Autodesk Inventor part; units mm, degrees
ref_plane "YZ Plane" through (0, 0, 0) normal (1, 0, 0) x (0, 1, 0)
ref_plane "XZ Plane" through (0, 0, 0) normal (0, 1, 0) x (-1, 0, 0)
ref_plane "XY Plane" through (0, 0, 0) normal (0, 0, 1) x (1, 0, 0)
ref_plane "Work Plane1" through (0, 0, -1.5) normal (0, 0, -1) x (-1, 0, 0)
sketch "Sketch1" plane through (0, 0, -1.5) normal (0, 0, -1) x (-1, 0, 0)
  line L0 (11.5, -60) -> (11.5, -65)
  arc A0 (9.3, -67.4819) -> (11.5, -65) centre (9, -65) ccw
  arc A1 (11.5, -60) -> (9.3, -57.5181) centre (9, -60) ccw
  line L1 (15, -75) -> (9.3, -75)
  line L2 (15, -5) -> (15, -75)
  line L3 (9.3, -5) -> (15, -5)
  line L4 (6.75, -60) -> (6.75, -65)
  arc A2 (6.75, -65) -> (11.25, -65) centre (9, -65) ccw
  line L5 (11.25, -65) -> (11.25, -60)
  arc A3 (11.25, -60) -> (6.75, -60) centre (9, -60) ccw
  line L6 (9, -65) -> (9, -61.5) construction
  line L7 (6.75, -65) -> (6.75, -61.5)
  line L8 (11.25, -61.5) -> (11.25, -65)
  arc A4 (6.75, -65) -> (11.25, -65) centre (9, -65) ccw
  arc A5 (11.25, -61.5) -> (6.75, -61.5) centre (9, -61.5) ccw
  line L9 (9.3, -57.5181) -> (9.3, -5)
  line L10 (9.3, -75) -> (9.3, -67.4819)
  point P0 (0, 0)
  point P1 (9, -63.25)
  dimension "d0" = 0.25
  dimension "d1" = 3.5
extrude "Extrusion1" add sketch "Sketch1" along normal blind 0.5 and the other way blind 1.5 contours A5 L5 A2 L4
sketch "Sketch2" plane through (0, 0, 0) normal (0, 0, 1) x (1, 0, 0)
  line L0 (-6.75, -65) -> (-6.75, -61.5)
  arc A0 (-6.75, -61.5) -> (-11.25, -61.5) centre (-9, -61.5) ccw
  line L1 (-11.25, -61.5) -> (-11.25, -65)
  arc A1 (-11.25, -65) -> (-6.75, -65) centre (-9, -65) ccw
  line L2 (-12.5, -69.5) -> (-5.5, -69.5)
  line L3 (-5.5, -69.5) -> (-5.5, -60.5)
  line L4 (-5.5, -60.5) -> (-12.5, -60.5)
  line L5 (-12.5, -60.5) -> (-12.5, -69.5)
  line L6 (-12.5, -69.5) -> (-5.5, -60.5) construction
  line L7 (-5.5, -69.5) -> (-12.5, -60.5) construction
  line L8 (-12.5, -57) -> (-5.5, -57)
  line L9 (-5.5, -57) -> (-5.5, -66)
  line L10 (-5.5, -66) -> (-12.5, -66)
  line L11 (-12.5, -66) -> (-12.5, -57)
  line L12 (-12.5, -57) -> (-5.5, -66) construction
  line L13 (-5.5, -57) -> (-12.5, -66) construction
  point P0 (0, 0)
  dimension "d6" = 7
  dimension "d7" = 7
  dimension "d9" = 9
extrude "Extrusion2" add sketch "Sketch2" along normal blind 1
ref_plane "Work Plane2" through (-10.6833, -67.2, 6.3) normal (-1, 0, 0) x (0, 0, 1)
sketch "Sketch3" plane through (-10.6833, -67.2, 6.3) normal (-1, 0, 0) x (0, 0, 1)
  line L0 (0.322, -0.2398) -> (-0.378, -0.2398)
  line L1 (-0.378, -1.4398) -> (-0.378, -0.2398)
  line L2 (-0.378, -1.4398) -> (0.322, -1.4398)
  line L3 (0.322, -1.4398) -> (0.322, -0.2398)
  line L4 (0.272, 0.6602) -> (-1.028, 0.6602)
  line L5 (-1.028, 0.6602) -> (-1.028, -2.3398)
  line L6 (-1.028, -2.3398) -> (0.272, -2.3398)
  line L7 (0.272, -2.3398) -> (0.272, 0.6602)
  line L8 (0.272, 0.6602) -> (-1.028, -2.3398) construction
  line L9 (-1.028, 0.6602) -> (0.272, -2.3398) construction
  line L10 (-1.028, -2.3398) -> (-5.3, -2.3398)
  line L11 (0.272, 0.6602) -> (-5.3, 3.95)
  line L12 (-5.3, -2.3) -> (-5.3, 10.2)
  line L13 (-5.3, 3.95) -> (-5.3, -2.3398)
  point P0 (-6.3, 67.2)
  point P1 (-0.378, -0.8398)
  point P2 (-5.3, -0.9)
  point P3 (0.272, -1.4398)
  point P4 (0.272, -0.2398)
  dimension "d12" = 1.3
  dimension "d13" = 3
extrude "Extrusion3" add sketch "Sketch3" along normal mid plane 2 contours L0 L1 L2 L7 L6 L5 L4 | L4 L5 L10 L13 L12 L11
sketch "Sketch4" plane through (-12.5, -69.5, 0) normal (0, -1, 0) x (1, 0, 0)
  point P0 (12.5, 0)
move faces "Move1" translate (0, 0, 0.5) faces at (-6.8944, -63.25, 1)
ref_plane "Work Plane3" through (-9.4833, -47.5, 19.3) normal (-1, 0, 0) x (0, 0, 1)
sketch "Sketch5" plane through (-11.6833, -69.5398, 6.572) normal (0, -1, 0) x (1, 0, 0)
  line L0 (2, 0) -> (0, 0)
  line L1 (0, -5.572) -> (0, 0)
  line L2 (2, -5.572) -> (0, -5.572)
  line L3 (2, 0) -> (2, -5.572)
  point P0 (11.6833, -6.572)
extrude "Extrusion4" cut sketch "Sketch5" against normal blind 7
move faces "Move3" translate (0, 0, -0.5) faces at (-6.8944, -63.0133, 1.5)
thicken "Thicken1" operation add thickness 0.5 both sides no extend neighbours yes toward (-1, 0, 0) faces at (-5.5, -65.3333, 0.6667)
thicken "Thicken2" operation add thickness 0.5 both sides no extend neighbours yes toward (1, 0, 0) faces at (-12.5, -61.1667, 0.3333)
thicken "Thicken3" operation add thickness 2 both sides no extend neighbours yes toward (0, -1, 0) faces at (-10, -69.5, 0.6667)
thicken "Thicken4" operation add thickness 1 both sides no extend neighbours yes toward (0, 1, 0) faces at (-8, -57, 0.3333)
move faces "Move4" translate (0, 0, -1) faces at (-9.75, -63.8333, -2)
sketch "Sketch6" plane through (-9, -65, -3) normal (0, 0, -1) x (-1, 0, 0)
  line L0 (-2.25, 3.5) -> (-2.25, 0)
  arc A0 (-2.25, 0) -> (2.25, 0) centre (0, 0) ccw
  line L1 (2.25, 0) -> (2.25, 3.5)
  arc A1 (2.25, 3.5) -> (-2.25, 3.5) centre (0, 3.5) ccw
  line L2 (-2.25, 3.5) -> (-2.25, 0)
  line L3 (2.25, 2.25) -> (-2.25, 2.25)
  line L4 (-2.25, 2.25) -> (-2.25, 1.25)
  line L5 (-2.25, 1.25) -> (2.25, 1.25)
  line L6 (2.25, 1.25) -> (2.25, 2.25)
  line L7 (2.25, 2.25) -> (-2.25, 1.25) construction
  line L8 (-2.25, 2.25) -> (2.25, 1.25) construction
  point P0 (-9, 65)
  point P1 (0, 1.75)
  point P2 (-2.25, 1.25)
  point P3 (2.25, 1.25)
  point P4 (2.25, 2.25)
  point P5 (-2.25, 2.25)
  dimension "d38" = 1
extrude "Extrusion5" cut sketch "Sketch6" against normal blind 1 contours L3 L1 L5 L0
fillet "Fillet1" radius 1 6 edges at (-6.75, -62.125, -3) (-11.25, -62.125, -3) (-9, -59.25, -3) (-11.25, -64.375, -3) (-6.75, -64.375, -3) (-9, -67.25, -3)
properties part number "switch_a"
For this review, take the finished solid that the model builds, in its own axes (mm). A direction names the side the tool comes from. Coordinates: 2 decimals unless noted, no trailing zeros. Order: outer loops, then holes, each group sorted by start corner. A loop starts at its lowest first (then second) coordinate and runs counter-clockwise, first axis right, second up. Notation, with made-up numbers: (-24, 31) - (13, 31) arc R24 cw to (13, 60) - close; hole circle Ø5 at (56.5, 9). An arc over 180 degrees is marked (long way). Answer as CSV lines item,"result". Start each with the question number.
1) Insertion check: P1, Ø2, axis at y = -63, z = -1.5, coming from the +X side; P2, Ø1, axis at y = -64, z = -1, coming from the -X side; P3, Ø0.8, axis at x = -8, z = -2.5, coming from the +Y side. Each pin has a flat end and moves straight along its axis. Give the tip position at first contact, or say it passes through.
2) Add section C-C (z = -1.2). State the section outline as (x, y) points, then the cut area to 3 significant figures.
3) Draft analysis for pull direction Y (two halves, no side actions). For faces 6 (the flat face through (-9, -71.5, 0.5)), 7 (the flat face through (-9, -63.75, -2.5)), 8 (the cylindrical face through (-10.949, -64.366, -2.715)), 9 (the flat face through (-9, -63, -2)), state which applies: +Y half, -Y half, draft (parallel to the pull), parting line (faces both ways), or undercut.
4) To check wall thickness, follow line 1 along Z through (x, y) = (-11.2, -59.75); line 2 along Z through (x, y) = (-10.8, -63.5); line 3 along Y through (x, z) = (-9.4, -2.2). State the ranges of each line that lie inside material, in increasing order. Write a range as [from, to].
5) Add section B-B (y = -57.5). State the section outline as (x, z) points, then the cut area to 3 significant figures.
6) Machinability: for faces 1 (the flat face through (-11.25, -63, -1)), 2 (the flat face through (-9, -62.75, -2.5)), 3 (the flat face through (-6.4, -63.6, 0)), 4 (the cylindrical face through (-8.95, -59.25, -0.99)), 5 (the cylindrical face through (-9.05, -67.25, -0.99)), which of the approach directions +Z, -Z, +X, -X, +Y, -Y give a long, thin tool a straight path to every point of the face, cutting with its end or side? Answer none if there is none.
7) Add section A-A (x = -9). State the section outline as (y, z) points.
Result:
1,P1,"x = -6.75"
1,P2,"x = -11.25"
1,P3,"y = -59.39"
2,outline,"(-11.25, -65) arc R2.25 ccw to (-6.75, -65) - (-6.75, -61.5) arc R2.25 ccw to (-11.25, -61.5) - close"
2,area,"31.7 mm^2"
3,face 6,"-Y half"
3,face 7,"undercut"
3,face 8,"draft"
3,face 9,"undercut"
4,line 1,"[0, 1]"
4,line 2,"[-2, 1]"
4,line 3,"[-67.19, -63.75], [-62.75, -59.31]"
5,outline,"(-12, 0) - (-6, 0) - (-6, 1) - (-12, 1) - close"
5,area,"6.00 mm^2"
6,face 1,"-Z, -X, +Y, -Y"
6,face 2,"-Z, +X, -X"
6,face 3,"-Z"
6,face 4,"-Z, +Y"
6,face 5,"-Z, -Y"
7,outline,"(-71.5, 0) - (-67.25, 0) - (-67.25, -2) arc R1 ccw to (-66.25, -3) - (-63.75, -3) - (-63.75, -2) - (-62.75, -2) - (-62.75, -3) - (-60.25, -3) arc R1 ccw to (-59.25, -2) - (-59.25, 0) - (-56, 0) - (-56, 1) - (-71.5, 1) - close"
